from build123d import *


with BuildPart() as f1:
    # F0 (on Front) → F1 (revolve)
    with BuildSketch(Plane.XZ):
        Polygon((24.319377, 61.028399), (0, 61.028399), (0, 23.788566), (67.676023, 23.788566), (67.676023, 37.304949), (44.225264, 37.304949), (44.225264, 48.212282), (24.319377, 48.212282), align=None)
        Polygon((0, 23.788566), (0, 61.028399), (-24.319377, 61.028399), (-24.319377, 48.212282), (-44.225264, 48.212282), (-44.225264, 37.304949), (-67.676023, 37.304949), (-67.676023, 23.788566), align=None)
    revolve(axis=Axis((2.036428, 0, 0), (-1, 0, 0)))


solid = f1.part
Work out the finished part from the listing and answer in its coordinate system (mm). A direction names the side the tool comes from. Give positions to 0.01 mm unless a question says otherwise; leave off trailing zeros. Order: outer loops, then holes, each group sorted by start corner. A loop starts at its lowest first (then second) coordinate and runs counter-clockwise, first axis right, second up. Notation, with made-up numbers: (45.25, 52) -> (90.25, 52) arc R17 cw to (90.25, 66) -> close; hole circle Ø6 at (-7, 23). An arc over 180 degrees is marked (long way). Answer as a JSON object with one key per item and string values. Group by question number.
1. Section A-A on z = 0 is taken. Determine the outline of the cut face in (x, y).
2. The mould has two halves that part along Y. Classify faces 1 (the cylindrical face through (0.947, -21.105, 10.977)), 2 (the flat face through (24.319, 18, -45)), 3 (the cylindrical face through (55.79, 1.64, -37.27)): released by +Y, released by -Y, zero draft, split by the parting line, or undercut.
3. Section D-D on y = 46 is taken. Determine the outline of the cut face in (x, z).
4. A tool of negligible diameter and unlimited length cuts with its end or side. For faces 4 (the cylindrical face through (-56.11, 1.64, -37.27)), 5 (the cylindrical face through (34.1, 47.8, -6.3)), 6 (the flat face through (-67.676, -24, -1)), from which of +Z, -Z, +X, -X, +Y, -Y can it reach the whole face along a straight path? Write none if from no direction.
5. Consider line 1 along Y through (x, z) = (15, 0); line 2 along Y through (x, z) = (37, 0); line 3 along X through (y, z) = (-4, -50). Determine where each line is inside the solid, lowest interval first. Write a range as [from, to].
6. Flat-ended cylindrical pins translate along their axes: pin 1 Ø8 at (x, y) = (44, -32.5) entering from +Z; pin 2 Ø1.5 at (x, y) = (21, 21.5) entering from -Z; pin 3 Ø6 at (x, z) = (-7.5, 45.5) entering from -Y. Find the tip coordinate at first contact, or state that the pin passes through.
7. Section C-C on x = 38 is taken. Determine the outline of the cut face in (y, z).
Result sheet:
{
 "1": {"outline": "(-67.68, -37.3) -> (-44.23, -37.3) -> (-44.23, -48.21) -> (-24.32, -48.21) -> (-24.32, -61.03) -> (24.32, -61.03) -> (24.32, -48.21) -> (44.23, -48.21) -> (44.23, -37.3) -> (67.68, -37.3) -> (67.68, -23.79) -> (-67.68, -23.79) -> close; (-67.68, 23.79) -> (67.68, 23.79) -> (67.68, 37.3) -> (44.23, 37.3) -> (44.23, 48.21) -> (24.32, 48.21) -> (24.32, 61.03) -> (-24.32, 61.03) -> (-24.32, 48.21) -> (-44.23, 48.21) -> (-44.23, 37.3) -> (-67.68, 37.3) -> close"},
 "2": {"face 1": "undercut", "face 2": "zero draft", "face 3": "split by the parting line"},
 "3": {"outline": "(-44.23, -14.44) -> (-24.32, -14.44) -> (-24.32, -40.11) -> (24.32, -40.11) -> (24.32, -14.44) -> (44.23, -14.44) -> (44.23, 14.44) -> (24.32, 14.44) -> (24.32, 40.11) -> (-24.32, 40.11) -> (-24.32, 14.44) -> (-44.23, 14.44) -> close"},
 "4": {"face 4": "-X", "face 5": "+X", "face 6": "+Z, -Z, -X, +Y, -Y"},
 "5": {"line 1": "y = [-61.03, -23.79], [23.79, 61.03]", "line 2": "y = [-48.21, -23.79], [23.79, 48.21]", "line 3": "x = [-24.32, 24.32]"},
 "6": {"pin 1": "stops at z = 38.89", "pin 2": "stops at z = -57.39", "pin 3": "stops at y = -43.8"},
 "7": {"outline": "circle Ø96.42 at (0, 0); hole circle Ø47.58 at (0, 0)"}
}
